```python
from build123d import *

# Parameters (mm, degrees)
SKETCH_2_W          = 50.043
SKETCH_2_H          = 47.687
EXTRUDE_1_DEPTH     = 1.6
SKETCH_3_R          = 1
CUT_EXTRUDE_1_DEPTH = 1.6
SKETCH_4_W          = 22.5
SKETCH_4_H          = 22.5
EXTRUDE_2_DEPTH     = 3
SKETCH_5_W          = 14.8
SKETCH_5_H          = 16.2
EXTRUDE_3_DEPTH     = 1.3
SKETCH_6_W          = 2.54
SKETCH_6_H          = 20.32
SKETCH_6_W_2        = 17.78
SKETCH_6_H_2        = 2.54
CUT_EXTRUDE_2_DEPTH = 0.1
SKETCH_7_W          = 6.5
SKETCH_7_H          = 6.5
EXTRUDE_4_DEPTH     = 1
SKETCH_8_R          = 2.75
EXTRUDE_5_DEPTH     = 8
SKETCH_9_R          = 2.1
CUT_EXTRUDE_3_DEPTH = 3


with BuildPart() as part:
    # 草图2 → 凸台-拉伸1 (new body)
    with BuildSketch(Plane(origin=(0, 0, 0), x_dir=(1, 0, 0), z_dir=(0, 1, 0))):
        Rectangle(SKETCH_2_W, SKETCH_2_H)
    extrude(amount=EXTRUDE_1_DEPTH)

    # 草图3 → 切除-拉伸1 (cut)
    with BuildSketch(Plane(origin=(0, 1.6, 0), x_dir=(1, 0, 0), z_dir=(0, 1, 0))):
        with Locations(Location((-22.75, 21.5, 0), (0, 0, 270))):
            Circle(SKETCH_3_R)
        with Locations(Location((22.75, 21.5, 0), (0, 0, 90))):
            Circle(SKETCH_3_R)
        with Locations(Location((22.75, -21.5, 0), (0, 0, 270))):
            Circle(SKETCH_3_R)
        with Locations(Location((-22.75, -21.5, 0), (0, 0, 90))):
            Circle(SKETCH_3_R)
    extrude(amount=-CUT_EXTRUDE_1_DEPTH, mode=Mode.SUBTRACT)

    # 草图4 → 凸台-拉伸2 (add)
    with BuildSketch(Plane(origin=(0, 1.6, 0), x_dir=(1, 0, 0), z_dir=(0, 1, 0))):
        with Locations((11.7715, -5.0935)):
            Rectangle(SKETCH_4_W, SKETCH_4_H)
    extrude(amount=EXTRUDE_2_DEPTH)

    # 草图5 → 凸台-拉伸3 (add)
    with BuildSketch(Plane(origin=(0, 1.6, 0), x_dir=(1, 0, 0), z_dir=(0, 1, 0))):
        with Locations((-15.9715, -11.1435)):
            Rectangle(SKETCH_5_W, SKETCH_5_H)
    extrude(amount=EXTRUDE_3_DEPTH)

    # 草图6 → 切除-拉伸2 (cut)
    with BuildSketch(Plane(origin=(0, 1.6, 0), x_dir=(1, 0, 0), z_dir=(0, 1, 0))):
        with Locations((-23.3715, 8.3165)):
            Rectangle(SKETCH_6_W, SKETCH_6_H)
        with Locations((9.3315, -22.0435)):
            Rectangle(SKETCH_6_W_2, SKETCH_6_H_2)
    extrude(amount=-CUT_EXTRUDE_2_DEPTH, mode=Mode.SUBTRACT)

    # 草图7 → 凸台-拉伸4 (add)
    with BuildSketch(Plane(origin=(0, 1.6, 0), x_dir=(1, 0, 0), z_dir=(0, 1, 0))):
        with Locations((10.9715, 19.5935)):
            Rectangle(SKETCH_7_W, SKETCH_7_H)
    extrude(amount=EXTRUDE_4_DEPTH)

    # 草图8 → 凸台-拉伸5 (add)
    with BuildSketch(Plane(origin=(0, 2.6, 0), x_dir=(1, 0, 0), z_dir=(0, 1, 0))):
        with Locations(Location((10.9715, 19.5935, 0), (0, 0, 270))):
            Circle(SKETCH_8_R)
    extrude(amount=EXTRUDE_5_DEPTH)

    # 草图9 → 切除-拉伸3 (cut)
    with BuildSketch(Plane(origin=(0, 10.6, 0), x_dir=(1, 0, 0), z_dir=(0, 1, 0))):
        with Locations(Location((10.9715, 19.5935, 0), (0, 0, 270))):
            Circle(SKETCH_9_R)
    extrude(amount=-CUT_EXTRUDE_3_DEPTH, mode=Mode.SUBTRACT)


solid = part.part
```
The model under review builds one solid part; all positions refer to its coordinate system, in mm. A direction names the side the tool comes from. Coordinates: 2 decimals unless noted, no trailing zeros. Write each loop counter-clockwise with the first axis right and the second up, starting at its lowest first coordinate (ties: lowest second). Pieces come first, ordered by that corner, then holes. Notation, with made-up numbers: (3.25, 2.5) -> (31.25, 2.5) arc R17 ccw to (31.25, 15.5) -> close; hole circle Ø6 at (11.25, 62). An arc over 180 degrees is marked (long way). One line per item, written item: value. Start each with the question number.
Q1. Add section C-C, the plane y = 3.5. Give the boundary of the cut face in (x, z), then the cut area to 3 significant figures.
Q2. The part is to be moulded in two halves that separate along Z. For faces 1 (the face through (-8.572, 2, 11)), 2 (the face through (-23.726, 0.811, -21.717)), 3 (the face through (12, 3, 16.343)), 4 (the face through (0, 1, -23.844)), say which applies: +Z half, -Z half, draft (parallel to the pull), parting line (faces both ways), or undercut.
Q3. For faces 5 (the face through (0.521, 3, 5)), 6 (the face through (9.694, 9.121, -21.26)), 7 (the face through (-16, 2, 3.044)), 8 (the face through (23.022, 3, 5)), 9 (the face through (-23.372, 2, 11)), list the 3-axis set-ups (+Z, -Z, +X, -X, +Y, -Y) from which the entire face can be reached by the end or side of a thin tool; tool diameter is ignored.
Q4. Add section D-D, the plane x = 19.5. Give the boundary of the cut face in (y, z).
Q5. To check wall thickness, follow probe 1 along X at (y, z) = (1, -21.5); probe 2 along X at (y, z) = (4, 2); probe 3 along Y at (x, z) = (-21.5, 10.5). State the ranges of each line that lie inside material, in increasing order.
Q6. Add section B-B, the plane z = 21.5. Give the boundary of the cut face in (x, y).
Q7. Clearance check with flat-ended pins moving along their axes: P1, Ø1.5, axis at x = 8.5, y = 7.5, coming from the -Z side; P2, Ø5, axis at y = 5, z = 3.5, coming from the +X side; P3, Ø3, axis at x = 11.5, z = 21.5, coming from the +Y side. State where each tip first meets the part, or that it passes through.
Q8. Add section A-A, the plane x = -22.75. Give the boundary of the cut face in (y, z), then the cut area to 3 significant figures.
Response:
1. outline: (0.52, -6.16) -> (23.02, -6.16) -> (23.02, 16.34) -> (0.52, 16.34) -> close; circle Ø5.5 at (10.97, -19.59)
1. area: 530 mm²
2. face 1: draft
2. face 2: undercut
2. face 3: +Z half
2. face 4: -Z half
3. face 5: +Z, -Z, +Y
3. face 6: +Y
3. face 7: -Z, -X, +Y
3. face 8: +Z, -Z, +X, +Y
3. face 9: +Z, -Z, -X, +Y
4. outline: (0, -23.84) -> (1.6, -23.84) -> (1.6, -6.16) -> (4.6, -6.16) -> (4.6, 16.34) -> (1.6, 16.34) -> (1.6, 23.84) -> (0, 23.84) -> close
5. probe 1: -25.02 to -23.75, -21.75 to 21.75, 23.75 to 25.02
5. probe 2: 0.52 to 23.02
5. probe 3: 0 to 2.9
6. outline: (-25.02, 0) -> (-23.75, 0) -> (-23.75, 1.6) -> (-25.02, 1.6) -> close; (-21.75, 0) -> (21.75, 0) -> (21.75, 1.6) -> (18.22, 1.6) -> (18.22, 1.5) -> (0.44, 1.5) -> (0.44, 1.6) -> (-21.75, 1.6) -> close; (23.75, 0) -> (25.02, 0) -> (25.02, 1.6) -> (23.75, 1.6) -> close
7. P1: z = -21.74
7. P2: x = 23.02
7. P3: y = 1.6
8. outline: (0, -23.84) -> (1.6, -23.84) -> (1.6, -22.5) -> (0, -22.5) -> close; (0, -20.5) -> (1.6, -20.5) -> (1.6, -18.48) -> (1.5, -18.48) -> (1.5, 1.84) -> (1.6, 1.84) -> (1.6, 3.04) -> (2.9, 3.04) -> (2.9, 19.24) -> (1.6, 19.24) -> (1.6, 20.5) -> (0, 20.5) -> close; (0, 22.5) -> (1.6, 22.5) -> (1.6, 23.84) -> (0, 23.84) -> close
8. area: 88.9 mm²
